Job drawing, mm, ordinate dimensions from the low corner. One solid piece. A direction names the side the tool comes from. Give positions to 0.01 mm unless a question says otherwise; leave off trailing zeros. Write each loop counter-clockwise with the first axis right and the second up, starting at its lowest first coordinate (ties: lowest second). Pieces come first, ordered by that corner, then holes. Notation, with made-up numbers: (17.25, -7.75) - (34.25, -7.75) arc R26 cw to (34.25, 21.25) - close; hole circle Ø9 at (51.5, 78). An arc over 180 degrees is marked (long way). Use a Markdown table: item, result. Add a question column.
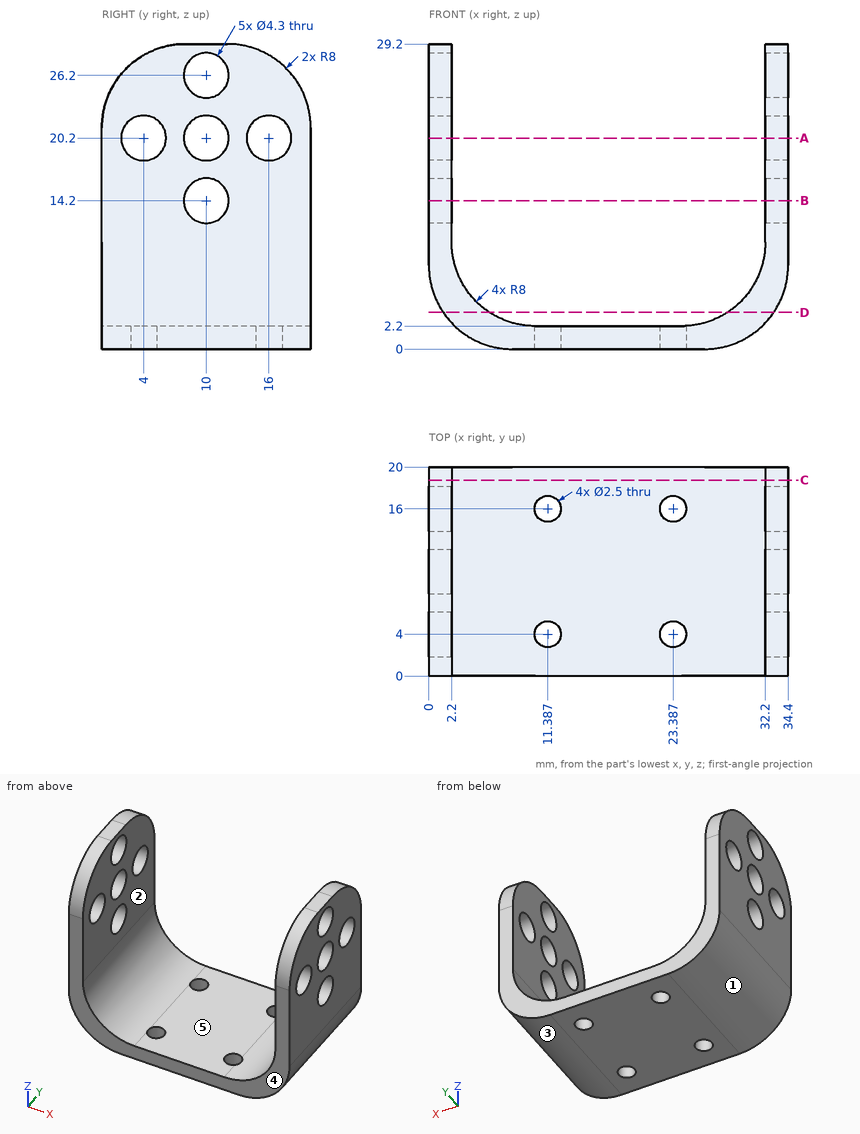
(1) Band-saw the part on C-C (y = 18.75). Write the cut outline in (x, z).
(2) Flat gauge pins, fed straight in: pin 1 (4 mm diameter, centred on x = 23.39, y = 4, fed in from -Z); pin 2 (3 mm diameter, centred on x = 11.39, y = 4, fed in from +Z); pin 3 (4 mm diameter, centred on y = 10, z = 20.2, fed in from -X); pin 4 (4 mm diameter, centred on x = 23.39, y = 16, fed in from +Z). Where does each tip first touch, or does it go through?
(3) Band-saw the part on D-D (z = 3.5). Write the cut outline in (x, y) (1 decimal), then the cut area to 3 significant figures.
(4) Which spindle directions (+Z, -Z, +X, -X, +Y, -Y) get a long thin tool onto all of the face, cutting with end or side? Do the marked faces 4 and 5. Say none if no direction does.
(5) Two-plate mould, pull along X, no slides. Class the marked faces 1, 2 and 3: +X half, -X half, draft (parallel to the pull), parting line (faces both ways), or undercut.
(6) Band-saw the part on B-B (z = 14.2). Write the cut outline in (x, y).
(7) Band-saw the part on A-A (z = 20.2). Give the number of separate pieces and of enclosed holes in the cut face.
(8) Probe probe 1 along Y at (x, z) = (33.35, 20.2); probe 2 along X at (y, z) = (9.75, 22.5); probe 3 along Z at (x, y) = (13.5, 2.75). List the from-to ranges inside material, lowest first. Write a range as [from, to].
Model answer:
| question | item | result |
|---|---|---|
| 1 | outline | (0, 8) arc R8 ccw to (8, 0) - (26.4, 0) arc R8 ccw to (34.4, 8) - (34.4, 25.49) - (32.2, 25.49) - (32.2, 10.2) arc R8 cw to (24.2, 2.2) - (10.2, 2.2) arc R8 cw to (2.2, 10.2) - (2.2, 25.49) - (0, 25.49) - close |
| 2 | pin 1 | stops at z = 0 |
| 2 | pin 2 | stops at z = 2.21 |
| 2 | pin 3 | passes through |
| 2 | pin 4 | stops at z = 2.29 |
| 3 | outline | (1.4, 0) - (5.8, 0) - (5.8, 20) - (1.4, 20) - close; (28.6, 0) - (33, 0) - (33, 20) - (28.6, 20) - close |
| 3 | area | 178 mm^2 |
| 4 | face 4 | +Z, -Z, +X, -X, -Y |
| 4 | face 5 | +Z, +Y, -Y |
| 5 | face 1 | -X half |
| 5 | face 2 | undercut |
| 5 | face 3 | +X half |
| 6 | outline | (0, 0) - (2.2, 0) - (2.2, 7.85) - (0, 7.85) - close; (0, 12.15) - (2.2, 12.15) - (2.2, 20) - (0, 20) - close; (32.2, 0) - (34.4, 0) - (34.4, 7.85) - (32.2, 7.85) - close; (32.2, 12.15) - (34.4, 12.15) - (34.4, 20) - (32.2, 20) - close |
| 7 | separate pieces | 8 |
| 7 | enclosed holes | 0 |
| 8 | probe 1 | y = [0, 1.85], [6.15, 7.85], [12.15, 13.85], [18.15, 20] |
| 8 | probe 2 | x = [0, 2.2], [32.2, 34.4] |
| 8 | probe 3 | z = [0, 2.2] |
